The drawing under review shows one solid part. Ordinate dimensions are in mm from its lowest x, y, z. A direction names the side the tool comes from. Round coordinates to 2 decimals unless told otherwise and drop trailing zeros. Loops run counter-clockwise (first coordinate to the right, second up) from the corner with the lowest first, then second, coordinate; pieces in that order, holes last. Notation, with made-up numbers: (28.25, -31.5) - (74.25, -31.5) arc R27 ccw to (74.25, -15.5) - close; hole circle Ø5 at (-28, 28). An arc over 180 degrees is marked (long way). Answer as CSV lines item,"result".
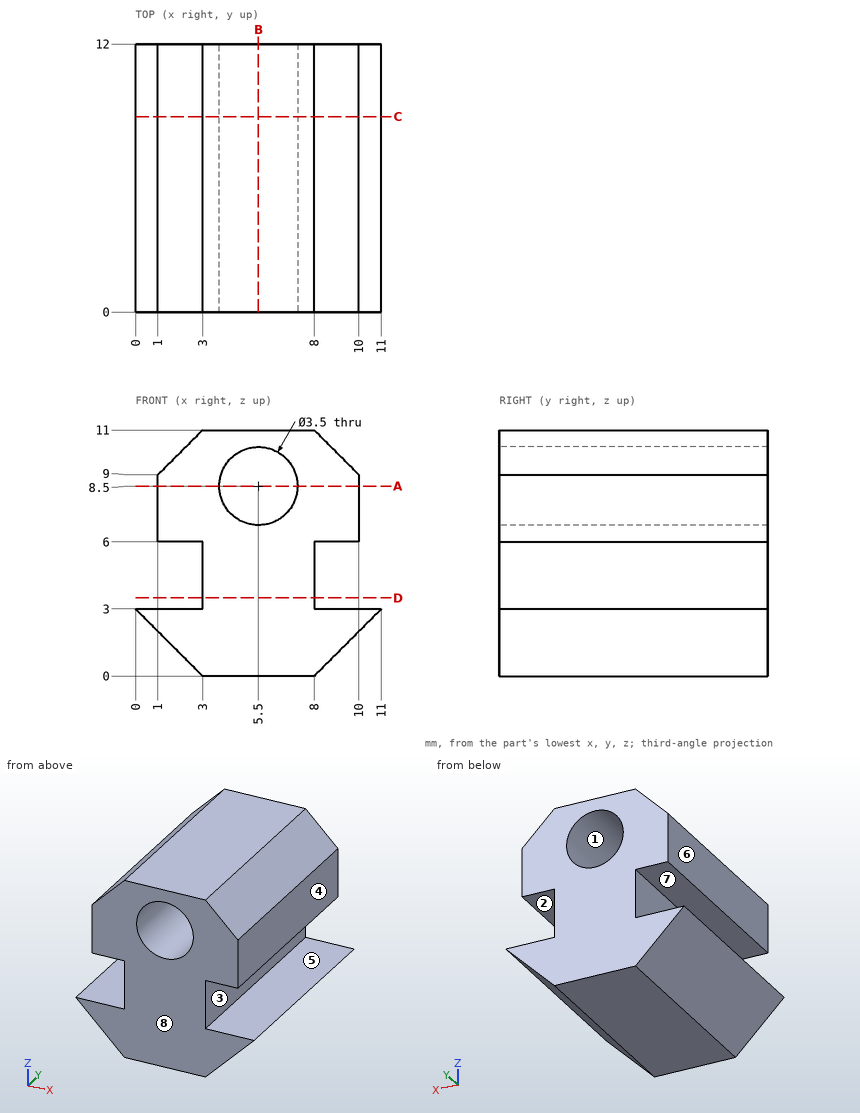
1. Take a section at A-A (z = 8.5). State the section outline as (x, y) points.
Numbers:
outline,"(1, 0) - (3.75, 0) - (3.75, 12) - (1, 12) - close; (7.25, 0) - (10, 0) - (10, 12) - (7.25, 12) - close"
2. Tool access review of the marked faces 4, 5, 6, 7 and 8: name each direction out of +Z, -Z, +X, -X, +Y, -Y from which nothing blocks a thin tool from reaching the whole face with its end or side.
Numbers:
face 4,"+Z, +X, +Y, -Y"
face 5,"+X, +Y, -Y"
face 6,"+Z, -X, +Y, -Y"
face 7,"-X, +Y, -Y"
face 8,"+Z, -Z, +X, -X, -Y"
3. Take a section at D-D (z = 3.5). State the section outline as (x, y) points, plus the area to 3 significant figures.
Numbers:
outline,"(3, 0) - (8, 0) - (8, 12) - (3, 12) - close"
area,"60.0 mm²"
4. Draft analysis for pull direction X (two halves, no side actions). For the marked faces 1, 2 and 3, state which applies: +X half, -X half, draft (parallel to the pull), parting line (faces both ways), or undercut.
Numbers:
face 1,"undercut"
face 2,"draft"
face 3,"+X half"
5. Take a section at C-C (y = 8.75). State the section outline as (x, z) points, plus the area to 3 significant figures.
Numbers:
outline,"(0, 3) - (3, 0) - (8, 0) - (11, 3) - (8, 3) - (8, 6) - (10, 6) - (10, 9) - (8, 11) - (3, 11) - (1, 9) - (1, 6) - (3, 6) - (3, 3) - close; hole circle Ø3.5 at (5.5, 8.5)"
area,"70.4 mm²"
6. Wall thickness on probe 1 along Z at (x, y) = (5.5, 6); probe 2 along Z at (x, y) = (2, 4.75); probe 3 along X at (y, z) = (4.25, 8.75): over which ranges is each line inside the solid? List them lowest first.
Numbers:
probe 1,"z = 0 to 6.75, 10.25 to 11"
probe 2,"z = 1 to 3, 6 to 10"
probe 3,"x = 1 to 3.77, 7.23 to 10"
7. Clearance check with flat-ended pins moving along their axes: pin 1 (2.5 mm diameter, centred on y = 5, z = 4, fed in from +X); pin 2 (0.6 mm diameter, centred on x = 2, y = 5, fed in from -Z); pin 3 (2.5 mm diameter, centred on y = 5.5, z = 8, fed in from -X). State where each tip first meets the part, or that it passes through.
Numbers:
pin 1,"stops at x = 11"
pin 2,"stops at z = 0.7"
pin 3,"stops at x = 1"
8. Take a section at B-B (x = 5.5). State the section outline as (y, z) points, plus the area to 3 significant figures.
Numbers:
outline,"(0, 0) - (12, 0) - (12, 6.75) - (0, 6.75) - close; (0, 10.25) - (12, 10.25) - (12, 11) - (0, 11) - close"
area,"90.0 mm²"
